from build123d import *

# Parameters (mm, degrees)
SKETCH1_R           = 2.25
SKETCH1_R_2         = 1.25282433
SKETCH1_W           = 40.6
SKETCH1_H           = 20.8
BOSS_EXTRUDE1_DEPTH = 3.175


with BuildPart() as part:
    # Sketch1 → Boss-Extrude1 (new body)
    with BuildSketch(Plane(origin=(0, 0, 0), x_dir=(1, 0, 0), z_dir=(0, 1, 0))):
        with BuildLine():
            Line((-162.38735588, 17.244652891), (-102.38735588, 17.244652891))
            Line((-102.38735588, 17.244652891), (7.61264412, 12.244652891))
            ThreePointArc((7.61264412, 12.244652891), (17.61264412, 2.244652891), (7.61264412, -7.755347109))
            Line((7.61264412, -7.755347109), (-102.38735588, -12.755347109))
            Line((-102.38735588, -12.755347109), (-162.38735588, -12.755347109))
            ThreePointArc((-162.38735588, -12.755347109), (-177.38735588, 2.244652891), (-162.38735588, 17.244652891))
        make_face()
        with Locations(Location((-168.38735588, 7.244652891, 0), (0, 0, 270))):
            Circle(SKETCH1_R, mode=Mode.SUBTRACT)
        with Locations(Location((-168.38735588, -2.755347109, 0), (0, 0, 270))):
            Circle(SKETCH1_R, mode=Mode.SUBTRACT)
        with Locations(Location((-118.78735588, 7.244652891, 0), (0, 0, 270))):
            Circle(SKETCH1_R, mode=Mode.SUBTRACT)
        with Locations(Location((-118.78735588, -2.755347109, 0), (0, 0, 270))):
            Circle(SKETCH1_R, mode=Mode.SUBTRACT)
        with Locations(Location((-42.38735588, 2.244652891, 0), (0, 0, 270))):
            Circle(SKETCH1_R, mode=Mode.SUBTRACT)
        with Locations(Location((3.23764412, 2.246310682, 0), (0, 0, 270))):
            Circle(SKETCH1_R_2, mode=Mode.SUBTRACT)
        with Locations((-142.392621679, 2.244652891)):
            Rectangle(SKETCH1_W, SKETCH1_H, mode=Mode.SUBTRACT)
    extrude(amount=BOSS_EXTRUDE1_DEPTH)


solid = part.part
Read the model definition and answer for the solid it produces. Units are mm, in the model's axes. A direction names the side the tool comes from. Give positions to 0.01 mm unless a question says otherwise; leave off trailing zeros. Loops run counter-clockwise (first coordinate to the right, second up) from the corner with the lowest first, then second, coordinate; pieces in that order, holes last. Notation, with made-up numbers: (46.25, 40.5) - (65.25, 40.5) arc R21 ccw to (65.25, 66.5) - close; hole circle Ø9 at (1.25, 74). An arc over 180 degrees is marked (long way). Answer as CSV lines item,"result". Start each with the question number.
1) Find section A-A (x = -136.5). Write down the section's boundary in (y, z) (3 decimals), then the cut area to 3 significant figures.
2) Each of these flat-tipped pins is pushed along its axis until it touches: pin 1 Ø1 at (y, z) = (1.5, -9.5) entering from -X; pin 2 Ø1.6 at (y, z) = (2, 1) entering from -X. Where does it stop, or does it pass through?
3) Find section B-B (y = 0.8). Write down the section's boundary in (x, z).
4) Determine the mould class of faces 1 (the face through (-116.557, 1.565, 2.462)), 2 (the face through (17.61, 1.57, -2.46)), 3 (the face through (-133, 2, -17.245)) for opening direction X: released by +X, released by -X, zero draft, split by the parting line, or undercut.
5) Straight lines are drawn through the part: L1, parallel to X at y = 3.05, z = 1.5; L2, parallel to X at y = 0.35, z = 2.5; L3, parallel to X at y = 2.25, z = -4. For each, find the intervals that lie inside material, in ascending order. Write a range as from..to.
6) Find section D-D (x = -74). Write down the section's boundary in (y, z) (3 decimals), then the cut area to 3 significant figures.
7) Find section C-C (z = -7). Write down the section's boundary in (x, y) (3 decimals).
8) Which of the six approach directions +Z, -Z, +X, -X, +Y, -Y give full straight-line access (tool end or side, diameter ignored) to faces 4 (the face through (-79, 0, -2)), 5 (the face through (-143, 2, -12.645))?
Findings below:
1,outline,"(0, -17.245) - (3.175, -17.245) - (3.175, -12.645) - (0, -12.645) - close; (0, 8.155) - (3.175, 8.155) - (3.175, 12.755) - (0, 12.755) - close"
1,area,"29.2 mm^2"
2,pin 1,"x = -175.78"
2,pin 2,"x = -177.19"
3,outline,"(-162.39, -17.24) - (-102.39, -17.24) - (7.61, -12.24) arc R10 ccw to (7.61, 7.76) - (-102.39, 12.76) - (-162.39, 12.76) arc R15 ccw to start; hole circle Ø4.5 at (-168.39, -7.24); hole circle Ø4.5 at (-168.39, 2.76); hole (-162.69, -12.64) - (-122.09, -12.64) - (-122.09, 8.16) - (-162.69, 8.16) - close; hole circle Ø4.5 at (-118.79, -7.24); hole circle Ø4.5 at (-118.79, 2.76); hole circle Ø4.5 at (-42.39, -2.24); hole circle Ø2.51 at (3.24, -2.25)"
4,face 1,"undercut"
4,face 2,"released by +X"
4,face 3,"zero draft"
5,L1,"-176.91..-170.25, -166.52..-162.69, -122.09..-120.65, -116.92..16.89"
5,L2,"-176.62..-170.62, -166.15..-162.69, -122.09..-121.02, -116.55..16.42"
5,L3,"-177.28..-162.69, -122.09..-43.79, -40.98..17.46"
6,outline,"(0, -15.954) - (3.175, -15.954) - (3.175, 11.465) - (0, 11.465) - close"
6,area,"87.1 mm^2"
7,outline,"(-176.614, 0) - (-170.624, 0) - (-170.624, 3.175) - (-176.614, 3.175) - close; (-166.151, 0) - (-162.693, 0) - (-162.693, 3.175) - (-166.151, 3.175) - close; (-122.093, 0) - (-121.024, 0) - (-121.024, 3.175) - (-122.093, 3.175) - close; (-116.551, 0) - (16.41, 0) - (16.41, 3.175) - (-116.551, 3.175) - close"
8,face 4,"+Z, -Z, +X, -X, -Y"
8,face 5,"+Y, -Y"
